The listing builds one solid part. Answer for the finished solid, in the listing's coordinates (mm). A direction names the side the tool comes from. Give positions to 0.01 mm unless a question says otherwise; leave off trailing zeros. Loops run counter-clockwise (first coordinate to the right, second up) from the corner with the lowest first, then second, coordinate; pieces in that order, holes last. Notation, with made-up numbers: (-12, 48.25) - (10, 48.25) arc R17 cw to (10, 77.25) - close; hole circle Ø5 at (25, 49). An arc over 180 degrees is marked (long way). Write each question's results on one line, items separated by ' | '.
from build123d import *

# Parameters (mm, degrees)
BOSS_EXTRUDE1_DEPTH                = 5
F_1_4_0_25_CLEARANCE_DOWEL_HOLE2_D = 6.499999954
SKETCH4_W                          = 12
SKETCH4_H                          = 20
BOSS_EXTRUDE2_DEPTH                = 48.5
SKETCH5_W                          = 20
SKETCH5_H                          = 10
CUT_EXTRUDE1_DEPTH                 = 7
F_4_0MM_CLEARANCE_DOWEL_HOLE1_D    = 4
CHAMFER1_SIZE                      = 7
FILLET1_R                          = 5


with BuildPart() as part:
    # Sketch1 → Boss-Extrude1 (new body)
    with BuildSketch(Plane(origin=(0, 0, 0), x_dir=(1, 0, 0), z_dir=(0, 1, 0))):
        Polygon((0, -10), (0, 10), (11.917176452, 10), (11.917176452, 32), (23.917176452, 32), (23.917176452, -32), (11.917176452, -32), (11.917176452, -10), align=None)
    extrude(amount=BOSS_EXTRUDE1_DEPTH)

    # 1/4 (0.25) Clearance Dowel Hole2 (through all)
    with Locations(Plane(origin=(0, 5, 0), x_dir=(1, 0, 0), z_dir=(0, 1, 0))):
        with Locations((17.917176452, -25.4), (17.917176452, 25.4)):
            Hole(F_1_4_0_25_CLEARANCE_DOWEL_HOLE2_D / 2)

    # Sketch4 → Boss-Extrude2 (add)
    with BuildSketch(Plane(origin=(0, 5, 0), x_dir=(1, 0, 0), z_dir=(0, 1, 0))):
        with Locations((6, 0)):
            Rectangle(SKETCH4_W, SKETCH4_H)
    extrude(amount=BOSS_EXTRUDE2_DEPTH)

    # Sketch5 → Cut-Extrude1 (cut)
    with BuildSketch(Plane.ZY):
        with Locations((0, 48.5)):
            Rectangle(SKETCH5_W, SKETCH5_H)
    extrude(amount=-CUT_EXTRUDE1_DEPTH, mode=Mode.SUBTRACT)

    # Ø4.0mm Clearance Dowel Hole1 (through all)
    with Locations(Plane.ZY.offset(-7)):
        with Locations((-5, 48.5), (5, 48.5)):
            Hole(F_4_0MM_CLEARANCE_DOWEL_HOLE1_D / 2)

    # Chamfer1
    chamfer1_edges = [part.edges().sort_by_distance(p)[0] for p in [
        (0, 43.5, 0),
    ]]
    chamfer(chamfer1_edges, length=CHAMFER1_SIZE - 0.0001)  # a hair under: the kernel refuses the full size

    # Fillet1
    fillet1_edges = [part.edges().sort_by_distance(p)[0] for p in [
        (11.917176452, 2.5, 10),
        (11.917176452, 2.5, -10),
        (0, 18.25005, 10),
        (0, 18.25005, -10),
    ]]
    fillet(fillet1_edges, radius=FILLET1_R)


solid = part.part
Item 1: For faces 4 (the face through (12, 29, 0)), 5 (the face through (18, 2, -32)), determine the directions among +Z, -Z, +X, -X, +Y, -Y from which every point of the face is accessible in a straight line to the end or side of a thin tool.
Values found:
face 4: +Z, -Z, +X, +Y | face 5: -Z, +X, -X, +Y, -Y
Item 2: A cutting plane is placed at B-B, the plane y = 48.5. Determine the outline of the cut face in (x, z), plus the area to 3 significant figures.
Values found:
outline: (7, -10) - (12, -10) - (12, -7) - (7, -7) - close; (7, -3) - (12, -3) - (12, 3) - (7, 3) - close; (7, 7) - (12, 7) - (12, 10) - (7, 10) - close | area: 60.0 mm²
Item 3: A cutting plane is placed at A-A, the plane z = -25.4. Determine the outline of the cut face in (x, y), plus the area to 3 significant figures.
Values found:
outline: (11.92, 0) - (14.67, 0) - (14.67, 5) - (11.92, 5) - close; (21.17, 0) - (23.92, 0) - (23.92, 5) - (21.17, 5) - close | area: 27.5 mm²
Item 4: Find the intervals of material crossed by line 1 along Y through (x, z) = (8.2, 5); line 2 along Z through (x, y) = (5, 40.5); line 3 along X through (y, z) = (2.95, 25.4), in increasing order. Write a range as [from, to].
Values found:
line 1: y = [0, 46.5], [50.5, 53.5] | line 2: z = [-10, 10] | line 3: x = [11.92, 14.67], [21.17, 23.92]
Item 5: For a pull along Y with two mould halves and no side action, classify faces 1 (the face through (7, 49, 0)), 2 (the face through (15, 0, 0)), 3 (the face through (9.535, 46.548, -4.566)) as released by +Y, released by -Y, zero draft, split by the parting line, or undercut.
Values found:
face 1: zero draft | face 2: released by -Y | face 3: undercut
Item 6: A cutting plane is placed at D-D, the plane y = 23. Determine the outline of the cut face in (x, z).
Values found:
outline: (0, -5) arc R5 ccw to (5, -10) - (12, -10) - (12, 10) - (5, 10) arc R5 ccw to (0, 5) - close
Item 7: Flat-ended cylindrical pins translate along their axes: P1, Ø5.5, axis at y = 1.5, z = -25, coming from the -X side; P2, Ø5, axis at x = 10.5, y = 43, coming from the -Z side; P3, Ø1, axis at y = 35.5, z = -8, coming from the +X side; P4, Ø3.5, axis at y = 48.5, z = -5, coming from the +X side. Find the tip coordinate at first contact, or state that the pin passes through.
Values found:
P1: stops at x = 11.92 | P2: stops at z = -10 | P3: stops at x = 12 | P4: passes through
